Can you work these out from the model? Positions are in its coordinate system, mm. A direction names the side the tool comes from. Coordinates: 2 decimals unless noted, no trailing zeros. Write each loop counter-clockwise with the first axis right and the second up, starting at its lowest first coordinate (ties: lowest second). Pieces come first, ordered by that corner, then holes.
Autodesk Inventor part; units mm, degrees
ref_plane "YZ Plane" through (0, 0, 0) normal (1, 0, 0) x (0, 1, 0)
ref_plane "XZ Plane" through (0, 0, 0) normal (0, 1, 0) x (-1, 0, 0)
ref_plane "XY Plane" through (0, 0, 0) normal (0, 0, 1) x (1, 0, 0)
sketch "Эскиз1" plane through (0, 0, 0) normal (0, 0, 1) x (1, 0, 0)
  line L0 (-54, -14) -> (54, -14)
  line L1 (54, -14) -> (54, 14)
  line L2 (54, 14) -> (-54, 14)
  line L3 (-54, 14) -> (-54, -14)
  line L4 (-54, -14) -> (54, 14) construction
  line L5 (54, -14) -> (-54, 14) construction
  point P0 (0, 0)
  dimension "d0" = 108
  dimension "d1" = 28
extrude "Выдавливание1" add sketch "Эскиз1" along normal blind 27.5
sketch "Эскиз2" plane through (0, 0, 27.5) normal (0, 0, 1) x (1, 0, 0)
  line L0 (-51, -11) -> (51, -11)
  line L1 (51, -11) -> (51, 11)
  line L2 (51, 11) -> (-51, 11)
  line L3 (-51, 11) -> (-51, -11)
  line L4 (-51, -11) -> (51, 11) construction
  line L5 (51, -11) -> (-51, 11) construction
  line L6 (54, 14) -> (-54, 14)
  line L7 (54, -14) -> (54, 14)
  point P0 (0, 0)
  dimension "d4" = 3
  dimension "d5" = 3
extrude "Выдавливание2" cut sketch "Эскиз2" against normal blind 24.5
sketch "Эскиз3" plane through (54, -14, 0) normal (1, 0, 0) x (0, 0, -1)
  line L0 (0, 28) -> (-27.5, 28)
  line L1 (0, 0) -> (-27.5, 0)
  line L2 (-27.5, 28) -> (-26, 28)
  line L3 (-26, 28) -> (-26, 0)
  line L4 (-26, 0) -> (-27.5, 0)
  line L5 (-27.5, 0) -> (-27.5, 28)
  point P0 (0, 14)
  dimension "d8" = 1.5
extrude "Выдавливание3" add sketch "Эскиз3" along normal blind 50
sketch "Эскиз4" plane through (0, 0, 27.5) normal (0, 0, 1) x (1, 0, 0)
  circle A0 centre (64, 0) radius 1.5
  line L0 (-54, -14) -> (104, -14)
  point P0 (0, 0)
  point P1 (54, -14)
  dimension "d11" = 3
  dimension "d12" = 14
  dimension "d13" = 10
extrude "Выдавливание4" cut sketch "Эскиз4" against normal blind 50
mirror "Зеркальное отражение1" about plane through (0, 0, 0) normal (1, 0, 0) of "Выдавливание3", "Выдавливание4"
sketch "Эскиз5" plane through (0, 0, 0) normal (0, 0, -1) x (-1, 0, 0)
  line L0 (-34, 4.1) -> (-25.8, 4.1)
  line L1 (-25.8, 4.1) -> (-25.8, -4.1)
  line L2 (-25.8, -4.1) -> (-34, -4.1)
  line L3 (-34, -4.1) -> (-34, 4.1)
  line L4 (-54, -14) -> (-54, 14)
  point P0 (0, 0)
  point P1 (-25.8, 0)
  dimension "d16" = 8.2
  dimension "d17" = 8.2
  dimension "d18" = 20
extrude "Выдавливание5" cut sketch "Эскиз5" against normal blind 10
equation "\"d16\" = d17"
properties part number "000.009 - Короб" material "Пластик АБС"
1. If we section it at A-A, the plane z = 9: List the corners of the cut face in (x, y) for me.
2. If I drill on L1, parallel to Y at x = 6, z = 25.75; L2, parallel to X at y = 8.5, z = 10; L3, parallel to Y at x = 64, z = 26.9, over which ranges is the centre line in solid material (lowest first)?
3. If we section it at C-C, the plane y = 9: List the corners of the cut face in (x, z) for me.
4. We'd pull the mould along Y, two halves only. Please class faces 5 (the face through (-1, 0, 3)), 6 (the face through (1, -14, 14)), 7 (the face through (-1, 0, 0)), 8 (the face through (-51, 0, 15)): released by +Y, released by -Y, zero draft, split by the parting line, or undercut.
5. I'm going to push flat-ended pins straight in: P1, Ø1.5, axis at y = -0.5, z = 1, coming from the -X side; P2, Ø1, axis at y = -1.5, z = 20.5, coming from the +X side; P3, Ø1.5, axis at x = 58.5, y = -5.5, coming from the -Z side. Where does each tip first touch, or does it pass through?
6. If we section it at B-B, the plane x = -5: List the corners of the cut face in (y, z) for me.
7. Which directions (+Z, -Z, +X, -X, +Y, -Y) give clear straight access to the entire face, cutting with the end or side of a thin tool? Please do faces 1 (the face through (79, 0, 26)), 2 (the face through (1, 14, 14)), 3 (the face through (1, 11, 15)), 4 (the face through (-79, 0, 26)).
Answers:
1. outline: (-54, -14) - (54, -14) - (54, 14) - (-54, 14) - close; hole (-51, -11) - (51, -11) - (51, 11) - (-51, 11) - close
2. L1: y = -14 to -11, 11 to 14
2. L2: x = -54 to -51, 51 to 54
2. L3: y = -14 to -1.5, 1.5 to 14
3. outline: (-104, 26) - (-54, 26) - (-54, 0) - (54, 0) - (54, 26) - (104, 26) - (104, 27.5) - (51, 27.5) - (51, 3) - (-51, 3) - (-51, 27.5) - (-104, 27.5) - close
4. face 5: undercut
4. face 6: released by -Y
4. face 7: zero draft
4. face 8: undercut
5. P1: stops at x = -54
5. P2: stops at x = 54
5. P3: stops at z = 26
6. outline: (-14, 0) - (14, 0) - (14, 27.5) - (11, 27.5) - (11, 3) - (-11, 3) - (-11, 27.5) - (-14, 27.5) - close
7. face 1: -Z, +X, +Y, -Y
7. face 2: +Z, -Z, +X, -X, +Y
7. face 3: +Z
7. face 4: -Z, -X, +Y, -Y
